Can you work these out from the model? Positions are in its coordinate system, mm. Give positions to 0.01 mm unless a question says otherwise; leave off trailing zeros. Write each loop counter-clockwise with the first axis right and the second up, starting at its lowest first coordinate (ties: lowest second). Pieces come first, ordered by that corner, then holes. Notation, with made-up numbers: (89.5, 0) -> (107.5, 0) arc R6 ccw to (107.5, 9) -> close; hole circle Ø5 at (67, 63.5). An arc over 180 degrees is marked (long way). One line per item, written item: value.
from build123d import *

# Parameters (mm, degrees)
ESQUISSE1_R        = 2.2
ESQUISSE1_R_2      = 1.7
BOSS_EXTRU_1_DEPTH = 4


with BuildPart() as part:
    # Esquisse1 → Boss.-Extru.1 (new body)
    with BuildSketch(Plane.XY):
        with BuildLine():
            Line((0, 10), (100, 10))
            ThreePointArc((100, 10), (110, 0), (100, -10))
            Line((100, -10), (0, -10))
            ThreePointArc((0, -10), (-10, 0), (0, 10))
        make_face()
        Circle(ESQUISSE1_R, mode=Mode.SUBTRACT)
        with Locations((100, 0)):
            Circle(ESQUISSE1_R, mode=Mode.SUBTRACT)
        with Locations((54.97928888, 4.178119463)):
            Circle(ESQUISSE1_R_2, mode=Mode.SUBTRACT)
        with Locations((45.02071112, -4.178119463)):
            Circle(ESQUISSE1_R_2, mode=Mode.SUBTRACT)
    extrude(amount=BOSS_EXTRU_1_DEPTH)


solid = part.part
1) We'd pull the mould along X, two halves only. Please class faces 1 (the face through (-10, 0, 2)), 2 (the face through (51, -10, 2)), 3 (the face through (97.802, 0.097, 1.972)): released by +X, released by -X, zero draft, split by the parting line, or undercut.
Answer list:
face 1: released by -X
face 2: zero draft
face 3: undercut
2) I need wall thicknesses on L1, parallel to Y at x = 55, z = 3.5; L2, parallel to X at y = -0.5, z = 0.45; L3, parallel to X at y = 4.75, z = 2.65. Which ranges of each line are inside material? Lowest first, please.
Answer list:
L1: y = -10 to 2.48, 5.88 to 10
L2: x = -9.99 to -2.14, 2.14 to 97.86, 102.14 to 109.99
L3: x = -8.8 to 53.38, 56.58 to 108.8
3) If we section it at A-A (y = 0): Write out the boundary of the cut face in (x, z), and give its area (3 significant figures).
Answer list:
outline: (-10, 0) -> (-2.2, 0) -> (-2.2, 4) -> (-10, 4) -> close; (2.2, 0) -> (97.8, 0) -> (97.8, 4) -> (2.2, 4) -> close; (102.2, 0) -> (110, 0) -> (110, 4) -> (102.2, 4) -> close
area: 445 mm^2
4) If we section it at C-C (y = -8.25): Write out the boundary of the cut face in (x, z), and give its area (3 significant figures).
Answer list:
outline: (-5.65, 0) -> (105.65, 0) -> (105.65, 4) -> (-5.65, 4) -> close
area: 445 mm^2
5) If we section it at B-B (z = 2.45): Write out the boundary of the cut face in (x, y).
Answer list:
outline: (0, -10) -> (100, -10) arc R10 ccw to (100, 10) -> (0, 10) arc R10 ccw to start; hole circle Ø4.4 at (0, 0); hole circle Ø3.4 at (45.02, -4.18); hole circle Ø3.4 at (54.98, 4.18); hole circle Ø4.4 at (100, 0)
6) Will these pins go through, and if not, where does the flat tip stop? pin 1 (2 mm diameter, centred on y = -2.5, z = 3, fed in from -X); pin 2 (3 mm diameter, centred on x = 45.02, y = -4.18, fed in from -Z).
Answer list:
pin 1: stops at x = -9.89
pin 2: passes through
